Autodesk Inventor part; units mm, degrees
ref_plane "YZ Plane" through (0, 0, 0) normal (1, 0, 0) x (0, 1, 0)
ref_plane "XZ Plane" through (0, 0, 0) normal (0, 1, 0) x (-1, 0, 0)
ref_plane "XY Plane" through (0, 0, 0) normal (0, 0, 1) x (1, 0, 0)
sketch "Boceto1" plane through (0, 0, 0) normal (0, 0, 1) x (1, 0, 0)
  line L0 (300, -450) -> (-300, -450)
  line L1 (-300, -450) -> (-300, 450)
  line L2 (-300, 450) -> (300, 450)
  line L3 (300, 450) -> (300, -450)
  line L4 (300, -450) -> (-300, 450) construction
  line L5 (-300, -450) -> (300, 450) construction
  line L6 (376.2, 526.2) -> (-376.2, 526.2)
  line L7 (-376.2, 526.2) -> (-376.2, -526.2)
  line L8 (-376.2, -526.2) -> (376.2, -526.2)
  line L9 (376.2, -526.2) -> (376.2, 526.2)
  line L10 (-300, -450) -> (-300, -526.2)
  line L11 (300, -450) -> (300, -526.2)
  line L12 (300, 450) -> (300, 526.2)
  line L13 (-300, 450) -> (-300, 526.2)
  line L14 (-300, -450) -> (-376.2, -450)
  line L15 (300, -450) -> (376.2, -450)
  point P0 (0, 0)
  dimension "d0" = 600
  dimension "d1" = 900
  dimension "d2" = 76.2
extrude "Extrusión1" add sketch "Boceto1" along normal blind 76.2 contours L11 L8 L10 L0 | L15 L9 L8 L11 | L3 L12 L6 L9 L15 | L14 L7 L6 L13 L1 | L10 L8 L7 L14 | L2 L13 L6 L12
extrude "Extrusión2" add sketch "Boceto1" along normal blind 1200 contours L15 L9 L8 L11 | L10 L8 L7 L14
sketch "Boceto2" plane through (300, -450, 76.2) normal (0, 1, 0) x (1, 0, 0)
  line L0 (76.2, 0) -> (76.2, -1123.8)
  line L1 (76.2, -1123.8) -> (76.2, -973.8)
  line L2 (76.2, -973.8) -> (0, -973.8)
  line L3 (0, 0) -> (0, -1123.8)
  line L4 (76.2, -973.8) -> (76.2, -897.6)
  line L5 (76.2, -897.6) -> (0, -897.6)
  line L6 (0, -897.6) -> (0, -973.8)
  line L7 (-600, 0) -> (-600, -1123.8)
  line L8 (-600, -897.6) -> (-600, -973.8)
  line L9 (-676.2, 0) -> (-676.2, -1123.8)
  line L10 (-676.2, -973.8) -> (-676.2, -897.6)
  line L11 (-600, -897.6) -> (-676.2, -897.6)
  line L12 (-600, -973.8) -> (-676.2, -973.8)
  point P0 (-300, 76.2)
  dimension "d7" = 150
  dimension "d8" = 76.2
extrude "Extrusión3" add sketch "Boceto2" along normal blind 350
sketch "Boceto3" plane through (376.2, -526.2, 0) normal (1, 0, 0) x (0, 0, -1)
  line L0 (0, 0) -> (0, 1052.4)
  line L1 (0, 1052.4) -> (-76.2, 1052.4)
  line L2 (-76.2, 76.2) -> (-76.2, 1052.4)
  line L3 (-76.2, 76.2) -> (-973.8, 76.2)
  line L4 (-973.8, 76.2) -> (-973.8, 426.2)
  line L5 (-1050, 426.2) -> (-973.8, 426.2)
  line L6 (-1050, 76.2) -> (-1050, 426.2)
  line L7 (-1050, 76.2) -> (-1200, 76.2)
  line L8 (-1200, 0) -> (-1200, 76.2)
  line L9 (0, 0) -> (-1200, 0)
  circle A0 centre (-1011.9, 375.4) radius 25.4
  line L10 (-1011.9, 375.4) -> (-1011.9, 426.2)
  line L11 (-973.8, 426.2) -> (-1050, 426.2)
  circle A1 centre (-1011.9, 375.4) radius 25.4
  circle A2 centre (-1011.9, 375.4) radius 33.4
  point P0 (0, 526.2)
  dimension "d11" = 50.8
  dimension "d12" = 50.8
  dimension "d16" = 8
extrude "Extrusión4" cut sketch "Boceto3" against normal blind 1200 contours A0
shell "Vaciado1" thickness 2 removed faces 2 at (325.4, -152.8439, 986.5824) at (-350.8, -152.8439, 986.5824)
extrude "Extrusión5" add sketch "Boceto3" against normal blind 76.2 contours A2
sketch "Boceto4" plane through (-376.2, -526.2, 0) normal (-1, 0, 0) x (0, 0, 1)
  circle A0 centre (1011.9, 375.4) radius 33.4
  circle A1 centre (1011.9, 375.4) radius 25.4
  point P0 (0, 526.2)
extrude "Extrusión6" add sketch "Boceto4" against normal blind 76.2
extrude "Extrusión7" add sketch "Boceto3" along normal blind 8.8 contours A2
extrude "Extrusión8" add sketch "Boceto4" along normal blind 8.8
sketch "Boceto5" plane through (376.2, -450, 973.8) normal (0, 0, -1) x (-1, 0, 0)
  point P0 (376.2, 450)
sketch "Boceto6" plane through (0, 0, 1200) normal (0, 0, 1) x (1, 0, 0)
  line L0 (374.2, -452) -> (302, -452)
  line L1 (302, -452) -> (302, -524.2)
  line L2 (374.2, -524.2) -> (374.2, -452)
  line L3 (302, -524.2) -> (374.2, -524.2)
  line L4 (300, -526.2) -> (376.2, -526.2)
  line L5 (300, -450) -> (300, -526.2)
  line L6 (300, -526.2) -> (376.2, -526.2)
  line L7 (376.2, -526.2) -> (376.2, -450)
  line L8 (376.2, -450) -> (300, -450)
  line L9 (-376.2, -450) -> (-376.2, -526.2)
  line L10 (-376.2, -526.2) -> (-300, -526.2)
  line L11 (-300, -526.2) -> (-300, -450)
  line L12 (-300, -450) -> (-376.2, -450)
  line L13 (-302, -452) -> (-374.2, -452)
  line L14 (-302, -524.2) -> (-302, -452)
  line L15 (-374.2, -452) -> (-374.2, -524.2)
  line L16 (-374.2, -524.2) -> (-302, -524.2)
  point P0 (0, 0)
extrude "Extrusión9" cut sketch "Boceto6" against normal blind 2 contours L2 L3 L1 L0 | L14 L16 L15 L13
sketch "Boceto7" plane through (300, -100, 76.2) normal (0, 1, 0) x (1, 0, 0)
  line L0 (-600, -973.8) -> (-600, -897.6)
  line L1 (-600, -897.6) -> (-676.2, -897.6)
  line L2 (-676.2, -897.6) -> (-676.2, -973.8)
  line L3 (-676.2, -973.8) -> (-600, -973.8)
  line L4 (-674.2, -899.6) -> (-674.2, -971.8)
  line L5 (-674.2, -971.8) -> (-602, -971.8)
  line L6 (-602, -899.6) -> (-674.2, -899.6)
  line L7 (-602, -971.8) -> (-602, -899.6)
  line L8 (0, -897.6) -> (0, -973.8)
  line L9 (0, -973.8) -> (76.2, -973.8)
  line L10 (76.2, -973.8) -> (76.2, -897.6)
  line L11 (76.2, -897.6) -> (0, -897.6)
  line L12 (2, -899.6) -> (2, -971.8)
  line L13 (2, -971.8) -> (74.2, -971.8)
  line L14 (74.2, -899.6) -> (2, -899.6)
  line L15 (74.2, -971.8) -> (74.2, -899.6)
  point P0 (-300, 76.2)
extrude "Extrusión10" cut sketch "Boceto7" against normal blind 2 contours L6 L7 L5 L4 | L14 L15 L13 L12
Check sheet for the modelled part. Datum: model origin and axes. Units: mm. A direction names the side the tool comes from. Round coordinates to 2 decimals unless told otherwise and drop trailing zeros. Loops run counter-clockwise (first coordinate to the right, second up) from the corner with the lowest first, then second, coordinate; pieces in that order, holes last. Notation, with made-up numbers: M 22.5,-13 L 72.5,-13 A25 ccw 72.5,24 Z; hole C 55,59.25 d11. An arc over 180 degrees is marked long. One line per question, with ' | ' between items. Start each with the question number.
Item 1: Gauge pin test, flat ends, axial feed: pin 1 Ø23 at (x, z) = (-333.5, 1157.5) entering from +Y; pin 2 Ø1.6 at (y, z) = (-101, 997.5) entering from -X; pin 3 Ø23 at (x, y) = (-330, -289.5) entering from -Z; pin 4 Ø23 at (x, z) = (-353.5, 1007) entering from +Y. Record the tip position at first contact, or that the pin passes through.
Item 2: Section check C-C (z = 693.5). Record the boundary of the cut face in (x, y), and give its area (3 significant figures).
Item 3: Section check D-D (x = 326.5). Record the boundary of the cut face in (y, z), and give its area (3 significant figures).
Item 4: Section check B-B (x = 159.5). Record the boundary of the cut face in (y, z).
Item 5: Scan lines: probe 1 along Y at (x, z) = (355.5, 1011.9); probe 2 along Z at (x, y) = (-318, -150); probe 3 along Y at (x, z) = (-382.25, 1011.9). Record each from-to range of solid material in increasing order.
Item 6: Section check A-A (y = -345). State how many separate pieces and enclosed holes the cut face has, and give its area (3 significant figures).
Item 7: Release check for a two-part mould opening along Y. For faces 1 (the face through (-338, 7, 2)), 2 (the face through (-341.1, -100, 1048.4)), 3 (the face through (339, -277, 1050)) record: released by +Y, released by -Y, zero draft, split by the parting line, or undercut.
Item 8: Set-up check for faces 4 (the face through (338, -450, 1124)), 5 (the face through (-4, 452, 38)), 6 (the face through (339, -277, 973.8)), 7 (the face through (338, -452, 519)): record each of +Z, -Z, +X, -X, +Y, -Y from which the full face is reachable in a straight line by a thin tool's end or side.
Worked out:
1) pin 1: y = -450 | pin 2: x = -376.2 | pin 3: z = 0 | pin 4: y = -117.4
2) outline: M -376.2,-526.2 L -300,-526.2 L -300,-450 L -376.2,-450 Z; M 300,-526.2 L 376.2,-526.2 L 376.2,-450 L 300,-450 Z; hole M -374.2,-524.2 L -302,-524.2 L -302,-452 L -374.2,-452 Z; hole M 302,-524.2 L 374.2,-524.2 L 374.2,-452 L 302,-452 Z | area: 1,190 mm^2
3) outline: M -526.2,0 L 526.2,0 L 526.2,76.2 L -450,76.2 L -450,973.8 L -100,973.8 L -100,975.8 L -452,975.8 L -452,74.2 L 524.2,74.2 L 524.2,2 L -524.2,2 L -524.2,1200 L -526.2,1200 Z; M -452,1048 L -100,1048 L -100,1050 L -450,1050 L -450,1200 L -452,1200 Z; C -150.8,1011.9 d66.8; hole C -150.8,1011.9 d50.8 | area: 11,600 mm^2
4) outline: M -526.2,0 L -450,0 L -450,76.2 L -526.2,76.2 Z; M 450,0 L 526.2,0 L 526.2,76.2 L 450,76.2 Z; hole M -524.2,2 L -452,2 L -452,74.2 L -524.2,74.2 Z; hole M 452,2 L 524.2,2 L 524.2,74.2 L 452,74.2 Z
5) probe 1: -526.2 to -524.2, -184.2 to -176.2, -125.4 to -117.4 | probe 2: 0 to 2, 74.2 to 76.2, 973.8 to 975.8, 978.51 to 986.51, 1037.29 to 1045.29, 1048 to 1050 | probe 3: -184.2 to -176.2, -125.4 to -117.4
6) separate pieces: 4 | enclosed holes: 4 | area: 2,370 mm^2
7) face 1: undercut | face 2: released by +Y | face 3: zero draft
8) face 4: +Z, +X, -X, +Y | face 5: none | face 6: +X, -X, +Y | face 7: +Z
